For this review, take the finished solid that the model builds, in its own axes (mm). Face numbers are marked on the shaded views. Give positions to 0.01 mm unless a question says otherwise; leave off trailing zeros. Write each loop counter-clockwise with the first axis right and the second up, starting at its lowest first coordinate (ties: lowest second). Pieces come first, ordered by that corner, then holes. Notation, with made-up numbers: M 80,26.5 L 92,26.5 A15 cw 92,54.5 Z; hole C 11,82 d9. An arc over 180 degrees is marked long. Write item = value, one per line.
Autodesk Inventor part; units mm, degrees
ref_plane "YZ Plane" through (0, 0, 0) normal (1, 0, 0) x (0, 1, 0)
ref_plane "XZ Plane" through (0, 0, 0) normal (0, 1, 0) x (-1, 0, 0)
ref_plane "XY Plane" through (0, 0, 0) normal (0, 0, 1) x (1, 0, 0)
sketch "Sketch1" plane through (0, 0, 0) normal (0, 1, 0) x (-1, 0, 0)
  line L0 (0, 0) -> (3.175, 0)
  line L1 (3.175, 0) -> (3.175, -3.175)
  line L2 (3.175, -3.175) -> (0, -3.175)
  line L3 (0, -3.175) -> (0, 0)
  line L4 (3.175, -3.175) -> (104.775, -3.175)
  line L5 (104.775, -3.175) -> (104.775, -94.615)
  line L6 (104.775, -94.615) -> (3.175, -94.615)
  line L7 (3.175, -94.615) -> (3.175, -3.175)
  line L8 (104.775, -94.615) -> (107.95, -94.615)
  line L9 (107.95, -94.615) -> (107.95, -97.79)
  line L10 (107.95, -97.79) -> (104.775, -97.79)
  line L11 (104.775, -97.79) -> (104.775, -94.615)
  line L12 (107.95, -97.79) -> (0, -97.79)
  line L13 (0, -97.79) -> (0, 0)
  line L14 (0, 0) -> (107.95, 0)
  line L15 (107.95, 0) -> (107.95, -97.79)
  dimension "d0" = 3.175
  dimension "d1" = 3.175
  dimension "d2" = 101.6
  dimension "d3" = 91.44
  dimension "d4" = 3.175
  dimension "d5" = 3.175
extrude "Extrusion1" add sketch "Sketch1" along normal blind 20 contours L0 L1 L2 L3 | L14 L15 L8 L5 L4 L1 | L2 L7 L6 L11 L12 L13 | L9 L10 L11 L8
sketch "Sketch6" plane through (0, 0, 0) normal (0, -1, 0) x (1, 0, 0)
  line L0 (-104.775, -3.175) -> (-3.175, -3.175)
  line L1 (-3.175, -3.175) -> (-3.175, -94.615)
  line L2 (-3.175, -94.615) -> (-104.775, -94.615)
  line L3 (-104.775, -94.615) -> (-104.775, -3.175)
  line L4 (0, 0) -> (0, -97.79)
  line L5 (-107.95, 0) -> (0, 0)
  line L6 (-107.95, -97.79) -> (-107.95, 0)
  line L7 (0, -97.79) -> (-107.95, -97.79)
extrude "Extrusion5" add sketch "Sketch6" against normal blind 3.175 contours L0 L1 L2 L3
sketch "Sketch7" plane through (0, 20, 0) normal (0, 1, 0) x (1, 0, 0)
  line L0 (-104.775, 3.175) -> (-3.175, 3.175)
  line L1 (-3.175, 3.175) -> (-3.175, 0)
  line L2 (-3.175, 0) -> (-104.775, 0)
  line L3 (-104.775, 0) -> (-104.775, 3.175)
  point P0 (0, 0)
extrude "Extrusion6" cut sketch "Sketch7" against normal blind 12.7
sketch "Sketch9" plane through (0, 3.175, 0) normal (0, 1, 0) x (1, 0, 0)
  line L0 (-104.775, 94.615) -> (-3.175, 94.615) construction
  line L1 (-104.775, 94.615) -> (-101.473, 94.615) construction
  line L2 (-101.473, 94.615) -> (-101.473, 89.535) construction
  line L3 (-101.473, 89.535) -> (-104.775, 89.535) construction
  line L4 (-104.775, 89.535) -> (-104.775, 94.615) construction
  line L5 (-3.175, 94.615) -> (-3.175, 3.175) construction
  line L6 (-101.473, 89.535) -> (-3.175, 89.535) construction
  line L7 (-3.175, 89.535) -> (-3.175, 3.175) construction
  line L8 (-3.175, 3.175) -> (-101.473, 3.175) construction
  line L9 (-101.473, 3.175) -> (-101.473, 89.535) construction
  line L10 (-101.473, 89.535) -> (-98.933, 89.535) construction
  line L11 (-98.933, 89.535) -> (-98.933, 85.725) construction
  line L12 (-98.933, 85.725) -> (-101.473, 85.725) construction
  line L13 (-101.473, 85.725) -> (-101.473, 89.535) construction
  line L14 (-3.175, 89.535) -> (-6.985, 89.535) construction
  line L15 (-6.985, 89.535) -> (-6.985, 85.725) construction
  line L16 (-6.985, 85.725) -> (-3.175, 85.725) construction
  line L17 (-3.175, 85.725) -> (-3.175, 89.535) construction
  circle A0 centre (-98.933, 85.725) radius 3.81
  circle A1 centre (-6.985, 85.725) radius 3.81
  point P0 (0, 0)
  dimension "d53" = 3.302
  dimension "d54" = 5.08
  dimension "d55" = 2.54
  dimension "d56" = 3.81
  dimension "d57" = 3.81
  dimension "d58" = 3.81
extrude "Extrusion9" add sketch "Sketch9" along normal blind 3.048
sketch "Sketch11" plane through (-104.775, 20, 0) normal (1, 0, 0) x (0, 0, -1)
  line L0 (89.535, -13.777) -> (81.915, -13.777)
  line L1 (85.725, -13.777) -> (62.103, -13.777)
  line L2 (62.103, -13.777) -> (62.103, -8.189)
  point P0 (0, -20)
  dimension "d103" = 5.588
hole "Hole3" at (-104.775, 11.811, -62.103) direction (-1, 0, 0) diameter 5.08 depth 4.064 tip angle 118
sketch "Sketch12" plane through (-98.933, 6.223, -85.725) normal (0, 1, 0) x (1, 0, 0)
  circle A0 centre (0, 0) radius 3.81
  circle A1 centre (91.948, 0) radius 3.81
  point P0 (98.933, -85.725)
  point P1 (95.758, 0)
hole "Hole4" at (-98.933, 6.223, -85.725) at (-6.985, 6.223, -85.725) direction (0, -1, 0) diameter 2.032 depth 4.064 tip angle 118
sketch "Sketch13" plane through (-104.775, 20, -94.615) normal (0, 0, 1) x (1, 0, 0)
  line L0 (9.652, -13.777) -> (2.032, -13.777)
  line L1 (5.842, -13.777) -> (19.304, -13.777)
  line L2 (19.304, -13.777) -> (19.304, -8.189)
  line L3 (19.304, -8.189) -> (28.194, -8.189)
  point P0 (104.775, -20)
  dimension "d84" = 13.462
  dimension "d85" = 5.588
  dimension "d86" = 8.89
hole "Hole5" at (-85.471, 11.811, -94.615) at (-76.581, 11.811, -94.615) direction (0, 0, -1) diameter 5.08 depth 4.064 tip angle 118
sketch "Sketch14" plane through (-104.775, 20, -94.615) normal (0, 0, 1) x (1, 0, 0)
  line L0 (0, -12.7) -> (101.6, -12.7)
  line L1 (101.6, -12.7) -> (101.6, -7.112)
  line L2 (101.6, -16.825) -> (101.6, 0)
  line L3 (101.6, -7.112) -> (86.36, -7.112)
  point P0 (104.775, -20)
  dimension "d94" = 5.588
  dimension "d95" = 15.24
hole "Hole6" at (-18.415, 12.888, -94.615) direction (0, 0, -1) diameter 7.62 depth 4.064 tip angle 118
sketch "Sketch15" plane through (0, 3.175, 0) normal (0, 1, 0) x (1, 0, 0)
  circle A0 centre (-98.933, 85.725) radius 1.016
  line L0 (-98.933, 85.725) -> (-86.233, 85.725)
  circle A1 centre (-6.985, 85.725) radius 1.016
  line L1 (-6.985, 85.725) -> (-19.685, 85.725)
  line L2 (-6.985, 85.725) -> (-6.985, 73.025)
  circle A2 centre (-98.933, 85.725) radius 3.81
  line L3 (-98.933, 85.725) -> (-98.933, 73.025)
  line L4 (-104.775, 3.175) -> (-95.7947, 12.1553)
  line L5 (-104.775, 3.175) -> (-92.075, 3.175) construction
  line L6 (-3.175, 85.725) -> (-3.175, 3.175)
  line L7 (-3.175, 3.175) -> (-12.1553, 12.1553)
  line L8 (-3.175, 3.175) -> (9.525, 3.175) construction
  line L9 (-98.933, 73.025) -> (-95.7947, 12.1553)
  line L10 (-104.775, 0) -> (-104.775, 94.615)
  line L11 (-95.7947, 12.1553) -> (-12.1553, 12.1553)
  line L12 (-12.1553, 12.1553) -> (-6.985, 73.025)
  line L13 (-6.985, 73.025) -> (-19.685, 85.725)
  line L14 (-19.685, 85.725) -> (-86.233, 85.725)
  line L15 (-86.233, 85.725) -> (-98.933, 73.025)
  line L16 (-104.775, 94.615) -> (-3.175, 94.615) construction
  line L17 (-53.975, 94.615) -> (-53.975, 3.175) construction
  line L18 (-104.775, 3.175) -> (-3.175, 3.175) construction
  line L19 (-53.975, 48.895) -> (-60.325, 48.895) construction
  line L20 (-60.325, 48.895) -> (-60.325, 55.245) construction
  line L21 (-60.325, 55.245) -> (-53.975, 55.245) construction
  line L22 (-53.975, 55.245) -> (-53.975, 48.895) construction
  line L23 (-53.975, 48.895) -> (-47.625, 48.895) construction
  line L24 (-47.625, 48.895) -> (-47.625, 42.545) construction
  line L25 (-47.625, 42.545) -> (-53.975, 42.545) construction
  line L26 (-53.975, 42.545) -> (-53.975, 48.895) construction
  line L27 (-86.233, 85.725) -> (-53.975, 55.245)
  line L28 (-53.975, 55.245) -> (-19.685, 85.725)
  line L29 (-6.985, 73.025) -> (-47.625, 48.895)
  line L30 (-98.933, 73.025) -> (-60.325, 48.895)
  line L31 (-3.175, 3.175) -> (-3.175, 15.875) construction
  line L32 (-3.175, 3.175) -> (-15.875, 3.175) construction
  line L33 (-11.3251, 21.9293) -> (-47.625, 48.895)
  line L34 (-24.9577, 12.1553) -> (-53.975, 42.545)
  line L35 (-104.775, 3.175) -> (-92.075, 3.175) construction
  line L36 (-104.775, 3.175) -> (-104.775, 15.875) construction
  line L37 (-96.3107, 22.1628) -> (-60.325, 48.895)
  line L38 (-53.975, 42.545) -> (-83.3844, 12.1553)
  point P0 (0, 0)
  dimension "d104" = 12.7
  dimension "d105" = 12.7
  dimension "d106" = 12.7
  dimension "d107" = 12.7
  dimension "d108" = 12.7
  dimension "d109" = 45
  dimension "d110" = 12.7
  dimension "d111" = 135
  dimension "d112" = 6.35
  dimension "d113" = 6.35
  dimension "d114" = 6.35
  dimension "d115" = 6.35
  dimension "d116" = 12.7
  dimension "d117" = 12.7
  dimension "d118" = 12.7
  dimension "d119" = 12.7
extrude "Extrusion10" cut sketch "Sketch15" against normal blind 25.4 contours L14 L28 L27 | L30 L37 L9 | L12 L33 L29 | L38 L34 L11
fillet "Fillet1" radius 3.175 12 edges at (-96.3107, 1.5875, -22.1628) (-60.325, 1.5875, -48.895) (-53.975, 1.5875, -55.245) (-53.975, 1.5875, -42.545) (-47.625, 1.5875, -48.895) (-83.3844, 1.5875, -12.1553) (-24.9577, 1.5875, -12.1553) (-86.233, 1.5875, -85.725) (-98.933, 1.5875, -73.025) (-19.685, 1.5875, -85.725) (-6.985, 1.5875, -73.025) (-11.3251, 1.5875, -21.9293)
sketch "Sketch16" plane through (0, 3.175, 0) normal (0, 1, 0) x (1, 0, 0)
  line L0 (-104.775, 3.175) -> (-104.775, 94.615) construction
  line L1 (-104.775, 94.615) -> (-85.725, 94.615) construction
  line L2 (-85.725, 94.615) -> (-85.725, 75.565) construction
  line L3 (-85.725, 75.565) -> (-104.775, 75.565) construction
  line L4 (-104.775, 75.565) -> (-104.775, 94.615) construction
  line L5 (-3.175, 94.615) -> (-22.225, 94.615) construction
  line L6 (-22.225, 94.615) -> (-22.225, 75.565) construction
  line L7 (-22.225, 75.565) -> (-3.175, 75.565) construction
  line L8 (-3.175, 75.565) -> (-3.175, 94.615) construction
  line L9 (-3.175, 3.175) -> (-104.775, 3.175) construction
  line L10 (-104.775, 3.175) -> (-92.075, 3.175) construction
  line L11 (-92.075, 3.175) -> (-92.075, 15.875) construction
  line L12 (-92.075, 15.875) -> (-104.775, 15.875) construction
  line L13 (-104.775, 15.875) -> (-104.775, 3.175) construction
  line L14 (-3.175, 3.175) -> (-15.875, 3.175) construction
  line L15 (-15.875, 3.175) -> (-15.875, 15.875) construction
  line L16 (-15.875, 15.875) -> (-3.175, 15.875) construction
  line L17 (-3.175, 15.875) -> (-3.175, 3.175) construction
  point P0 (0, 0)
  dimension "d123" = 19.05
  dimension "d124" = 19.05
  dimension "d125" = 19.05
  dimension "d126" = 19.05
  dimension "d127" = 12.7
  dimension "d128" = 12.7
  dimension "d129" = 12.7
  dimension "d130" = 12.7
hole "Hole7" at (-3.175, 3.175, -94.615) at (-85.725, 3.175, -75.565) at (-22.225, 3.175, -75.565) at (-15.875, 3.175, -15.875) at (-92.075, 3.175, -15.875) direction (0, -1, 0) diameter 3.175 depth 25.4 tip angle 118
properties part number "radiocase" material "ABS Plastic"
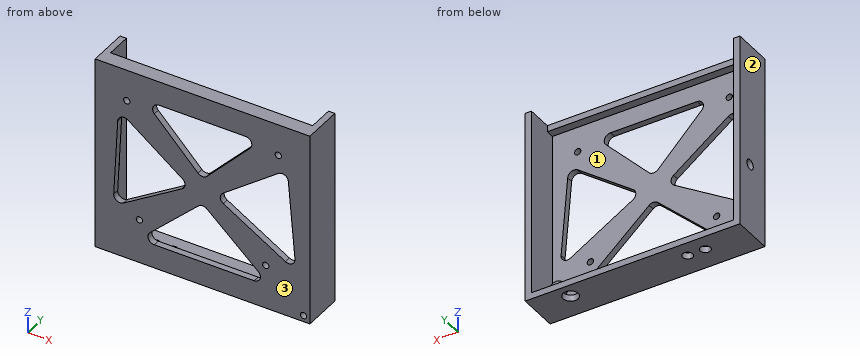
1. We need section B-B, the plane y = 5. Write out the cut boundary in (x, z) (3 decimals).
Responses:
outline = M -107.95,-97.79 L 0,-97.79 L 0,0 L -107.95,0 Z; C -98.933,-85.725 d7.62; C -6.985,-85.725 d7.62; hole M -104.775,-94.615 L -3.175,-94.615 L -3.175,-3.175 L -104.775,-3.175 Z; hole C -98.933,-85.725 d2.032; hole C -6.985,-85.725 d2.032
2. We need section D-D, the plane x = -58. Write out the cut boundary in (y, z) (3 decimals), then the cut area to 3 significant figures.
Responses:
outline = M 0,-97.79 L 20,-97.79 L 20,-94.615 L 3.175,-94.615 L 3.175,-85.725 L 0,-85.725 Z; M 0,-59.048 L 3.175,-59.048 L 3.175,-38.386 L 0,-38.386 Z; M 0,-12.155 L 3.175,-12.155 L 3.175,-3.175 L 7.3,-3.175 L 7.3,0 L 0,0 Z
area = 209 mm2
3. The part is to be moulded in two halves that separate along X. For the marked faces 1, 2 and 3, say which applies: +X half, -X half, draft (parallel to the pull), parting line (faces both ways), or undercut.
Responses:
face_1 = undercut
face_2 = -X half
face_3 = draft
4. We need section A-A, the plane x = -39. Write out the cut boundary in (y, z) (3 decimals).
Responses:
outline = M 0,-97.79 L 20,-97.79 L 20,-94.615 L 3.175,-94.615 L 3.175,-85.725 L 0,-85.725 Z; M 0,-68.556 L 3.175,-68.556 L 3.175,-54.016 L 0,-54.016 Z; M 0,-42.488 L 3.175,-42.488 L 3.175,-26.862 L 0,-26.862 Z; M 0,-12.155 L 3.175,-12.155 L 3.175,-3.175 L 7.3,-3.175 L 7.3,0 L 0,0 Z
5. We need section C-C, the plane z = -83.5. Write out the cut boundary in (x, y) (3 decimals), then the cut area to 3 significant figures.
Responses:
outline = M -107.95,0 L -81.279,0 L -81.279,3.175 L -95.84,3.175 L -95.84,6.223 L -102.026,6.223 L -102.026,3.175 L -104.775,3.175 L -104.775,20 L -107.95,20 Z; M -25.006,0 L 0,0 L 0,20 L -3.175,20 L -3.175,3.175 L -3.892,3.175 L -3.892,6.223 L -10.078,6.223 L -10.078,3.175 L -25.006,3.175 Z
area = 309 mm2
6. Insertion check: P1, Ø2.5, axis at x = -56.5, z = -2, coming from the +Y side; P2, Ø1, axis at x = -2.5, z = -94.5, coming from the -Y side (3 decimals); P3, Ø3, axis at y = 11.811, z = -62.103, coming from the -X side (3 decimals). Each pin has a flat end and moves straight along its axis. Give the tip position at first contact, or say it passes through.
Responses:
P1 = 7.3
P2 = 3.175
P3 = -3.175
7. For line 1 along X through (y, z) = (8, -16.5) (3 decimals); line 2 along X through (y, z) = (1.25, -67); line 3 along Z through (x, y) = (-50, 4.75) (3 decimals), list the stretches that pass through material, from the lowest coordinate up. Write a range as from..to.
Responses:
line_1 = -107.95..-104.775, -3.175..0
line_2 = -107.95..-98.62, -89.29..-66.42, -40.75..-17.13, -7.5..0
line_3 = -97.79..-94.615, -3.175..0
